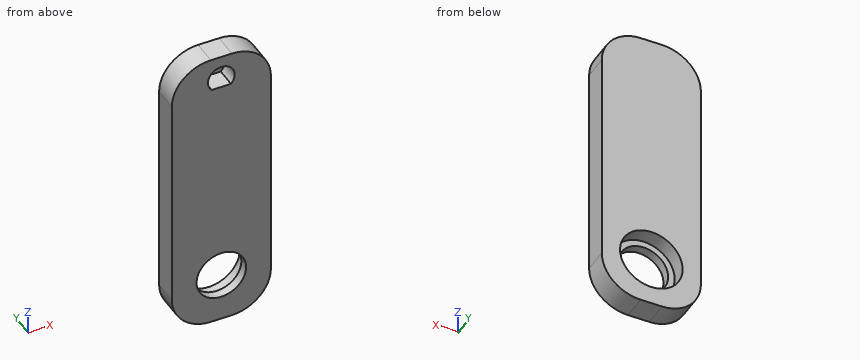
```python
from build123d import *

# Parameters (mm, degrees)
SKETCH1_W           = 25.4
SKETCH1_H           = 76.2
BOSS_EXTRUDE1_DEPTH = 6.35
SKETCH5_R           = 8.016875
CUT_EXTRUDE1_DEPTH  = 3.96875
SKETCH6_R           = 6.35
CUT_EXTRUDE2_DEPTH  = 81.419841933
SKETCH7_R           = 3.429
CUT_EXTRUDE3_DEPTH  = 7.62
SKETCH9_W           = 11.198432991
SKETCH9_H           = 1.819618823
BOSS_EXTRUDE2_DEPTH = 6.35
BOSS_EXTRUDE4_START = -6.35
SKETCH11_W          = 13.636513595
SKETCH11_H          = 8.31497605
BOSS_EXTRUDE4_DEPTH = 1.27
FILLET1_R           = 10


with BuildPart() as part:
    # Sketch1 → Boss-Extrude1 (new body)
    with BuildSketch(Plane(origin=(0, 0, 0), x_dir=(1, 0, 0), z_dir=(0, 1, 0))):
        with Locations((12.7, 38.1)):
            Rectangle(SKETCH1_W, SKETCH1_H)
    extrude(amount=BOSS_EXTRUDE1_DEPTH)

    # Sketch5 → Cut-Extrude1 (cut)
    with BuildSketch(Plane(origin=(0, 6.35, 0), x_dir=(1, 0, 0), z_dir=(0, 1, 0))):
        with Locations(Location((12.7, 63.5, 0), (0, 0, 270))):
            Circle(SKETCH5_R)
    extrude(amount=-CUT_EXTRUDE1_DEPTH, mode=Mode.SUBTRACT)

    # Sketch6 → Cut-Extrude2 (cut, through all)
    with BuildSketch(Plane(origin=(0, 2.38125, 0), x_dir=(1, 0, 0), z_dir=(0, 1, 0))):
        with Locations(Location((12.7, 63.5, 0), (0, 0, 270))):
            Circle(SKETCH6_R)
    extrude(amount=-CUT_EXTRUDE2_DEPTH, mode=Mode.SUBTRACT)

    # Sketch7 → Cut-Extrude3 (cut)
    with BuildSketch(Plane(origin=(0, 6.35, 0), x_dir=(1, 0, 0), z_dir=(0, 1, 0))):
        with Locations(Location((12.7, 6.35, 0), (0, 0, 270))):
            Circle(SKETCH7_R)
    extrude(amount=-CUT_EXTRUDE3_DEPTH, mode=Mode.SUBTRACT)

    # Sketch9 → Boss-Extrude2 (add, through all)
    with BuildSketch(Plane(origin=(0, 6.35, 0), x_dir=(1, 0, 0), z_dir=(0, 1, 0))):
        with Locations((12.325928429, 9.647409411)):
            Rectangle(SKETCH9_W, SKETCH9_H)
    extrude(amount=-BOSS_EXTRUDE2_DEPTH)

    # Sketch11 → Boss-Extrude4 (add)
    with BuildSketch(Plane.XZ.offset(BOSS_EXTRUDE4_START)):
        with Locations((12.44089651, -6.12924614)):
            Rectangle(SKETCH11_W, SKETCH11_H)
    extrude(amount=BOSS_EXTRUDE4_DEPTH)

    # Fillet1
    fillet1_edges = [part.edges().sort_by_distance(p)[0] for p in [
        (0, 3.175, -76.2),
        (25.4, 3.175, -76.2),
        (25.4, 3.175, 0),
        (0, 3.175, 0),
    ]]
    fillet(fillet1_edges, radius=FILLET1_R)


solid = part.part
```
CAD build for the part. Positions are in the model's coordinates, mm. Coordinates: 2 decimals unless noted, no trailing zeros. Write each loop counter-clockwise with the first axis right and the second up, starting at its lowest first coordinate (ties: lowest second). Pieces come first, ordered by that corner, then holes.
(1) Flat gauge pins, fed straight in: pin 1 (1.5 mm diameter, centred on x = 6.5, z = -63.5, fed in from +Y); pin 2 (1.5 mm diameter, centred on x = 21.5, y = 2.5, fed in from -Z). Where does each tip first touch, or does it go through?
(2) Cut at D-D, the plane x = 8. List the corners of the cut face in (y, z).
(3) Drill centre lines: probe 1 along X at (y, z) = (0.8, -63.5); probe 2 along X at (y, z) = (4.2, -63.5); probe 3 along Z at (x, y) = (9.75, 5.75). Where is each one in solid material? Low to high.
(4) Cut at B-B, the plane y = 0.75. List the corners of the cut face in (x, z), and give its area (3 significant figures).
(5) Cut at A-A, the plane x = 12.7. List the corners of the cut face in (y, z).
(6) Cut at C-C, the plane z = -63.5. List the corners of the cut face in (x, y), and give its area (3 significant figures).
Geometry says:
1. pin 1: stops at y = 2.38
1. pin 2: stops at z = -74.65
2. outline: (0, -76) - (6.35, -76) - (6.35, -69.99) - (2.38, -69.99) - (2.38, -67.77) - (0, -67.77) - close; (0, -59.23) - (2.38, -59.23) - (2.38, -57.01) - (6.35, -57.01) - (6.35, -0.2) - (0, -0.2) - close
3. probe 1: x = 0 to 6.35, 19.05 to 25.4
3. probe 2: x = 0 to 4.68, 20.72 to 25.4
3. probe 3: z = -76.2 to -70.95, -56.05 to 0
4. outline: (0, -66.2) arc R10 ccw to (10, -76.2) - (15.4, -76.2) arc R10 ccw to (25.4, -66.2) - (25.4, -10) arc R10 ccw to (15.4, 0) - (10, 0) arc R10 ccw to (0, -10) - close; hole circle Ø12.7 at (12.7, -63.5); hole (10.24, -8.74) - (15.16, -8.74) arc R3.43 ccw (long way) to start
4. area: 1,690 mm2
5. outline: (0, -76.2) - (6.35, -76.2) - (6.35, -71.52) - (2.38, -71.52) - (2.38, -69.85) - (0, -69.85) - close; (0, -57.15) - (2.38, -57.15) - (2.38, -55.48) - (6.35, -55.48) - (6.35, 0) - (0, 0) - (0, -2.92) - (5.08, -2.92) - (5.08, -8.74) - (0, -8.74) - close
6. outline: (0, 0) - (6.35, 0) - (6.35, 2.38) - (4.68, 2.38) - (4.68, 6.35) - (0, 6.35) - close; (19.05, 0) - (25.4, 0) - (25.4, 6.35) - (20.72, 6.35) - (20.72, 2.38) - (19.05, 2.38) - close
6. area: 67.4 mm2
